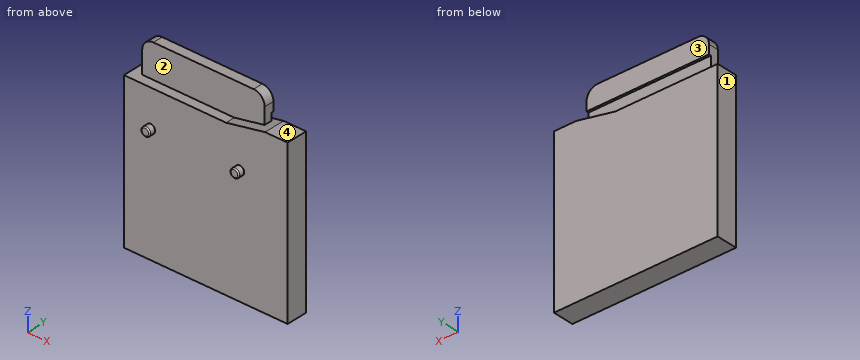
from build123d import *

# Parameters (mm, degrees)
SKETCH1_W               = 14.7
SKETCH1_H               = 14.5
BOSS_EXTRUDE1_DEPTH     = 1.9
CUT_EXTRUDE1_DEPTH      = 1
CUT_EXTRUDE1_DEPTH_BACK = 1.9
SKETCH3_W               = 11
SKETCH3_H               = 0.7
BOSS_EXTRUDE2_DEPTH     = 3
SKETCH4_W               = 11
SKETCH4_H               = 1.8
BOSS_EXTRUDE3_DEPTH     = 0.2
FILLET1_R               = 1
SKETCH5_R               = 0.4
BOSS_EXTRUDE4_DEPTH     = 0.55
FILLET2_R               = 0.1


with BuildPart() as part:
    # Sketch1 → Boss-Extrude1 (new body)
    with BuildSketch(Plane(origin=(0, 0, 0), x_dir=(1, 0, 0), z_dir=(0, 1, 0))):
        Rectangle(SKETCH1_W, SKETCH1_H)
    extrude(amount=BOSS_EXTRUDE1_DEPTH)

    # Sketch2 → Cut-Extrude1 (cut, two sides)
    with BuildSketch(Plane(origin=(0, 1.9, 0), x_dir=(1, 0, 0), z_dir=(0, 1, 0))) as cut_extrude1_sk:
        Polygon((-57.675178239, -6.55), (-7.35, -6.55), (1.824899914, -6.55), (5.328458875, -7.25), (54.6782833, -17.109938843), (45.259811524, -117.318654275), (-67.093650016, -106.758715432), align=None)
    extrude(amount=CUT_EXTRUDE1_DEPTH, mode=Mode.SUBTRACT)
    extrude(cut_extrude1_sk.sketch, amount=-CUT_EXTRUDE1_DEPTH_BACK, mode=Mode.SUBTRACT)

    # Sketch3 → Boss-Extrude2 (add)
    with BuildSketch(Plane.XY.offset(6.55)):
        with Locations((-0.95, 1.2)):
            Rectangle(SKETCH3_W, SKETCH3_H)
    extrude(amount=BOSS_EXTRUDE2_DEPTH)

    # Sketch4 → Boss-Extrude3 (add)
    with BuildSketch(Plane(origin=(0, 1.55, 0), x_dir=(1, 0, 0), z_dir=(0, 1, 0))):
        with Locations((-0.95, -8.65)):
            Rectangle(SKETCH4_W, SKETCH4_H)
    extrude(amount=BOSS_EXTRUDE3_DEPTH)

    # Fillet1
    fillet1_edges = [part.edges().sort_by_distance(p)[0] for p in [
        (-6.45, 1.3, 9.55),
        (4.55, 1.3, 9.55),
    ]]
    fillet(fillet1_edges, radius=FILLET1_R)

    # Sketch5 → Boss-Extrude4 (add)
    with BuildSketch(Plane.XZ):
        with Locations((-4.95, 3.25)):
            Circle(SKETCH5_R)
        with Locations((3.05, 3.25)):
            Circle(SKETCH5_R)
    extrude(amount=BOSS_EXTRUDE4_DEPTH)

    # Fillet2
    fillet2_edges = [part.edges().sort_by_distance(p)[0] for p in [
        (-5.35, -0.55, 3.25),
        (2.65, -0.55, 3.25),
    ]]
    fillet(fillet2_edges, radius=FILLET2_R)


solid = part.part
The listing builds one solid part. Answer for the finished solid, in the listing's coordinates (mm). Face numbers are marked on the shaded views. A direction names the side the tool comes from. Round coordinates to 2 decimals unless told otherwise and drop trailing zeros. Order: outer loops, then holes, each group sorted by start corner. A loop starts at its lowest first (then second) coordinate and runs counter-clockwise, first axis right, second up. Notation, with made-up numbers: (66.25, -28.75) -> (115.25, -28.75) arc R30 ccw to (115.25, -5.75) -> close; hole circle Ø4 at (39, 88.5). An arc over 180 degrees is marked (long way). Write each question's results on one line, items separated by ' | '. Start each with the question number.
Q1. Which of the six approach directions +Z, -Z, +X, -X, +Y, -Y give full straight-line access (tool end or side, diameter ignored) to the marked faces 1, 2, 3 and 4?
Q2. Find section B-B (z = 3.25). Determine the outline of the cut face in (x, y).
Q3. Each of these flat-tipped pins is pushed along its axis until it touches: pin 1 (1 mm diameter, centred on x = 6.5, y = 0.5, fed in from +Z); pin 2 (0.7 mm diameter, centred on y = 1, z = 8, fed in from -X); pin 3 (2 mm diameter, centred on x = -1, z = 8.5, fed in from +Y). Where does it stop, or does it pass through?
Q4. Find section C-C (x = -4.95). Determine the outline of the cut face in (y, z), then the cut area to 3 significant figures.
Q5. Find section D-D (y = -0.2). Determine the outline of the cut face in (x, z).
Q6. Straight lines are drawn through the part: probe 1 along Z at (x, y) = (-3.25, 1.7); probe 2 along Y at (x, z) = (-0.25, -5.5); probe 3 along Z at (x, y) = (6.5, 0.2). For each, find the intervals that lie inside material, in ascending order. Write a range as from..to.
Q7. Find section A-A (y = 1.2). Determine the outline of the cut face in (x, z), then the cut area to 3 significant figures.
Worked answers:
1) face 1: +Z, -Z, -X, +Y, -Y | face 2: +Z, -X, -Y | face 3: +Z, +X, -X, +Y | face 4: +Z, +X, +Y, -Y
2) outline: (-7.35, 0) -> (-5.35, 0) -> (-5.35, -0.45) arc R0.1 ccw to (-5.25, -0.55) -> (-4.65, -0.55) arc R0.1 ccw to (-4.55, -0.45) -> (-4.55, 0) -> (2.65, 0) -> (2.65, -0.45) arc R0.1 ccw to (2.75, -0.55) -> (3.35, -0.55) arc R0.1 ccw to (3.45, -0.45) -> (3.45, 0) -> (7.35, 0) -> (7.35, 1.9) -> (-7.35, 1.9) -> close
3) pin 1: stops at z = 7.25 | pin 2: stops at x = -6.45 | pin 3: stops at y = 1.75
4) outline: (-0.55, 2.95) arc R0.1 ccw to (-0.45, 2.85) -> (0, 2.85) -> (0, -7.25) -> (1.9, -7.25) -> (1.9, 6.55) -> (1.55, 6.55) -> (1.55, 7.75) -> (1.75, 7.75) -> (1.75, 9.55) -> (0.85, 9.55) -> (0.85, 6.55) -> (0, 6.55) -> (0, 3.65) -> (-0.45, 3.65) arc R0.1 ccw to (-0.55, 3.55) -> close | area: 29.1 mm2
5) outline: circle Ø0.8 at (-4.95, 3.25); circle Ø0.8 at (3.05, 3.25)
6) probe 1: z = -7.25..6.55, 7.75..9.55 | probe 2: y = 0..1.9 | probe 3: z = -7.25..7.25
7) outline: (-7.35, -7.25) -> (7.35, -7.25) -> (7.35, 7.25) -> (5.33, 7.25) -> (4.55, 7.09) -> (4.55, 8.55) arc R1 ccw to (3.55, 9.55) -> (-5.45, 9.55) arc R1 ccw to (-6.45, 8.55) -> (-6.45, 6.55) -> (-7.35, 6.55) -> close | area: 237 mm2
